Autodesk Inventor part; units mm, degrees
ref_plane "YZ Plane" through (0, 0, 0) normal (1, 0, 0) x (0, 1, 0)
ref_plane "XZ Plane" through (0, 0, 0) normal (0, 1, 0) x (-1, 0, 0)
ref_plane "XY Plane" through (0, 0, 0) normal (0, 0, 1) x (1, 0, 0)
sketch "Sketch1" plane through (0, 0, 0) normal (0, 0, 1) x (1, 0, 0)
  line L0 (-25.4, -25.4) -> (25.4, -25.4)
  line L1 (25.4, -25.4) -> (25.4, 25.4)
  line L2 (25.4, 25.4) -> (-25.4, 25.4)
  line L3 (-25.4, 25.4) -> (-25.4, -25.4)
  line L4 (-25.4, -25.4) -> (25.4, 25.4) construction
  line L5 (25.4, -25.4) -> (-25.4, 25.4) construction
  point P0 (0, 0)
  dimension "d0" = 50.8
extrude "Extrusion1" add sketch "Sketch1" along normal mid plane 25.4
ref_plane "Work Plane1" through (0, 0, 9.525) normal (0, 0, 1) x (1, 0, 0)
sketch "Sketch2" plane through (0, 0, 9.525) normal (0, 0, 1) x (1, 0, 0)
  arc A0 (0, -6.985) -> (0, 6.985) centre (0, 0) ccw
  line L0 (0, -6.985) -> (0, 6.985)
  dimension "d5" = 6.985
revolve "Revolution1" cut sketch "Sketch2" angle 360 about axis through (0, -6.985, 9.525) along (0, 1, 0)
equation "\"d0\" = sideLength"
equation "\"d1\" = partDepth"
equation "\"d5\" = radiusofBallHole"
equation "\"d3\" = -workPlaneForBallDistanceFfromFontEdge"
equation "\"radiusofBallHole\" = 0.5 * diameterOfBallHole"
equation "\"sideLength\" = 50.8"
equation "\"partDepth\" = 25.4"
equation "\"workPlaneForBallDistanceFfromFontEdge\" = 3.175"
equation "\"allowancForBallToRotate\" = 1.27"
properties part number "socket"
CAD build for the part. Positions are in the model's coordinates, mm. Coordinates: 2 decimals unless noted, no trailing zeros. Order: outer loops, then holes, each group sorted by start corner. A loop starts at its lowest first (then second) coordinate and runs counter-clockwise, first axis right, second up. Notation, with made-up numbers: (44.5, -33.75) -> (51.5, -33.75) arc R19 ccw to (51.5, -13.75) -> close; hole circle Ø5 at (31, 37.25). An arc over 180 degrees is marked (long way). Use one line per item in the form item = value. Start each with the question number.
1) Band-saw the part on D-D on z = 11.5. Give the cut face in (x, y).
2) Drill centre lines: L1, parallel to Z at x = -22.5, y = 23; L2, parallel to X at y = -3, z = 9.25; L3, parallel to X at y = 1, z = 12. Where is each one in solid material? Low to high. Write a range as [from, to].
3) Band-saw the part on C-C on z = 5.75. Give the cut face in (x, y).
4) Band-saw the part on A-A on x = -15. Give the cut face in (y, z), then the cut area to 3 significant figures.
5) Drop a flat-ended pin along its axis: pin 1 (1 mm diameter, centred on x = 4.5, y = -7.5, fed in from +Z). Give the stop position or say it passes through.
Entries:
q1.outline = (-25.4, -25.4) -> (25.4, -25.4) -> (25.4, 25.4) -> (-25.4, 25.4) -> close; hole circle Ø13.4 at (0, 0)
q2.L1 = [-12.7, 12.7]
q2.L2 = [-25.4, -6.3], [6.3, 25.4]
q2.L3 = [-25.4, -6.45], [6.45, 25.4]
q3.outline = (-25.4, -25.4) -> (25.4, -25.4) -> (25.4, 25.4) -> (-25.4, 25.4) -> close; hole circle Ø11.75 at (0, 0)
q4.outline = (-25.4, -12.7) -> (25.4, -12.7) -> (25.4, 12.7) -> (-25.4, 12.7) -> close
q4.area = 1,290 mm2
q5.pin_1 = 12.7
